from build123d import *

# Parameters (mm, degrees)
SALIENTE_EXTRUIR1_DEPTH = 3


with BuildPart() as part:
    # Model → Saliente-Extruir1 (new body)
    with BuildSketch(Plane.XY):
        with BuildLine():
            Line((57.876051331, 16.193461244), (57.893981077, 40.180349578))
            Line((57.893981077, 40.180349578), (57.893981077, 50.180349578))
            Line((57.893981077, 50.180349578), (49.867941077, 50.180349578))
            Line((49.867941077, 50.180349578), (49.867941077, 31.597099578))
            Line((49.867941077, 31.597099578), (49.867941077, 14.013849578))
            ThreePointArc((49.867941077, 14.013849578), (52.233805345, 9.208034607), (57.367941077, 7.680349578))
            ThreePointArc((57.367941077, 7.680349578), (59.6653644, 6.596184281), (62.200359504, 6.430751104))
            ThreePointArc((62.200359504, 6.430751104), (62.9704791, 6.972225641), (62.949576341, 7.913417408))
            ThreePointArc((62.949576341, 7.913417408), (62.082712456, 8.936213823), (60.897352842, 9.562702519))
            ThreePointArc((60.897352842, 9.562702519), (62.218292049, 9.458452731), (63.516644878, 9.723081417))
            ThreePointArc((63.516644878, 9.723081417), (64.2274431, 10.680349578), (63.516644878, 11.637617739))
            ThreePointArc((63.516644878, 11.637617739), (61.945301969, 11.880701786), (60.367941077, 11.680349578))
            ThreePointArc((60.367941077, 11.680349578), (61.630469791, 12.22740936), (62.779023795, 12.985087958))
            ThreePointArc((62.779023795, 12.985087958), (63.087813038, 14.136299223), (62.075412289, 14.765332526))
            ThreePointArc((62.075412289, 14.765332526), (60.636782457, 14.535665244), (59.249346326, 14.091341219))
            ThreePointArc((59.249346326, 14.091341219), (58.409082944, 14.132037192), (57.897205789, 14.799630249))
            ThreePointArc((57.897205789, 14.799630249), (57.815004717, 15.495458697), (57.876051331, 16.193461244))
        make_face()
    extrude(amount=SALIENTE_EXTRUIR1_DEPTH)


solid = part.part
Input: part model. Units: mm. Frame: model coordinates. A direction names the side the tool comes from. Give positions to 0.01 mm unless a question says otherwise; leave off trailing zeros. Order: outer loops, then holes, each group sorted by start corner. A loop starts at its lowest first (then second) coordinate and runs counter-clockwise, first axis right, second up. Notation, with made-up numbers: (-4, 69.5) -> (5, 69.5) arc R11 ccw to (5, 82.5) -> close; hole circle Ø9 at (19.5, 2.5). An arc over 180 degrees is marked (long way). Use one line per item in the form item = value.
1) Section B-B, the plane y = 43. Return loops of the section in (x, z).
Response values:
outline = (49.87, 0) -> (57.89, 0) -> (57.89, 3) -> (49.87, 3) -> close
2) First-contact query: pin 1 Ø1 at (y, z) = (23, 1.5) entering from +X; pin 2 Ø6 at (x, y) = (52, 21) entering from -Z; pin 3 Ø1.5 at (x, z) = (54, 0.5) entering from -Y. Flat tips, straight axial feed; report the tip coordinate or a pass-through.
Response values:
pin_1 = 57.88
pin_2 = 0
pin_3 = 7.88
3) Section C-C, the plane x = 54. Return loops of the section in (y, z), and give its area (3 significant figures).
Response values:
outline = (8.13, 0) -> (50.18, 0) -> (50.18, 3) -> (8.13, 3) -> close
area = 126 mm^2
4) Mould query, pull axis Y, two halves, no side actions, for faces 1 (the cylindrical face through (63.1, 14.1, 1.5)), 2 (the cylindrical face through (52.175, 9.258, 1.479)), 3 (the cylindrical face through (58.42, 14.126, 1.479)). Classes: pulls with the +Y half, pulls with the -Y half, needs draft (parallel to the pull), parting line crosses it, or undercut.
Response values:
face_1 = undercut
face_2 = pulls with the -Y half
face_3 = pulls with the +Y half
5) Section A-A, the plane z = 2.2. Return loops of the section in (x, y), and give its area (3 significant figures).
Response values:
outline = (49.87, 14.01) arc R6.69 ccw to (57.37, 7.68) arc R6.8 ccw to (62.2, 6.43) arc R1 ccw to (62.95, 7.91) arc R3.54 ccw to (60.9, 9.56) arc R4.75 ccw to (63.52, 9.72) arc R1 ccw to (63.52, 11.64) arc R5.7 ccw to (60.37, 11.68) arc R7.91 ccw to (62.78, 12.99) arc R1 ccw to (62.08, 14.77) arc R9.62 ccw to (59.25, 14.09) arc R1 cw to (57.9, 14.8) arc R3.43 cw to (57.88, 16.19) -> (57.89, 40.18) -> (57.89, 50.18) -> (49.87, 50.18) -> close
area = 371 mm^2
6) Line query: probe 1 along Y at (x, z) = (61.5, 1.5); probe 2 along Y at (x, z) = (62.5, 0.25); probe 3 along Y at (x, z) = (56.5, 0.8). Output: solid intervals per line, ascending.
Response values:
probe_1 = 6.38 to 9.32, 9.47 to 11.87, 12.16 to 14.7
probe_2 = 6.52 to 8.54, 9.48 to 11.85, 12.77 to 14.71
probe_3 = 7.63 to 50.18
7) Reachability of faces 4 (the flat face through (54, 50.18, 1)), 5 (the cylindrical face through (60.66, 14.54, 1.48)) from +Z, -Z, +X, -X, +Y, -Y: full face, straight path, thin tool, end or side. Return the list, or none.
Response values:
face_4 = +Z, -Z, +X, -X, +Y
face_5 = +Z, -Z, +Y
